Geometry check sheet. Reference: the model listing, model coordinates, mm. Face numbers are marked on the shaded views. Coordinates: 2 decimals unless noted, no trailing zeros. Order: outer loops, then holes, each group sorted by start corner. A loop starts at its lowest first (then second) coordinate and runs counter-clockwise, first axis right, second up. Notation, with made-up numbers: (1, 6.25) - (21, 6.25) arc R24 cw to (21, 40.25) - close; hole circle Ø1 at (-36, -7). An arc over 180 degrees is marked (long way). Use CSV: the item, a comma, the result in double quotes. Start each with the question number.
1) Sectioned sample at A-A, the plane y = 2.3. Record the cut outline in (x, z).
2) Sectioned sample at D-D, the plane x = 41.5. Count the separate pieces of the cut face and the enclosed holes in it, and give its area (3 significant figures).
3) Sectioned sample at C-C, the plane z = 6. Record the cut outline in (x, y), and give its area (3 significant figures).
4) Thickness scan on probe 1 along Z at (x, y) = (47, 2.15); probe 2 along Y at (x, z) = (48, 13); probe 3 along Z at (x, y) = (41, -0.4). Record the ranges inside material, lowest first. Write a range as [from, to].
5) Depth check by flat-ended pin: P1, Ø0.8, axis at y = -0.5, z = 6.5, coming from the +X side; P2, Ø17, axis at x = 36.5, z = 28.5, coming from the +Y side; P3, Ø3, axis at y = 0.5, z = 17, coming from the -X side. Enter the tip coordinate at first touch or a pass-through.
6) Sectioned sample at B-B, the plane x = 47. Record the cut outline in (y, z).
7) Draft check along Z on the marked faces 1 and 2. Enter one of: released by +Z, released by -Z, zero draft, split by the parting line, or undercut.
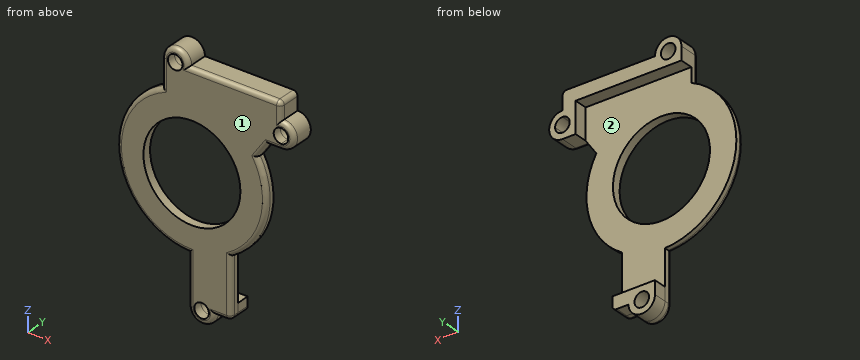
from build123d import *

# Parameters (mm, degrees)
F0_R     = 11
F1_DEPTH = 2
F2_DEPTH = 3
F3_R     = 1


with BuildPart() as f1:
    # F0 (on Front) → F1 (new body)
    with BuildSketch(Plane.XZ):
        with BuildLine():
            Line((38, 47), (38, 44))
            Line((38, 44), (62, 44))
            Line((62, 44), (62, 37))
            Line((62, 37), (65, 37))
            Line((65, 37), (65, 38.35))
            ThreePointArc((65, 38.35), (63.35, 40), (65, 41.65))
            Line((65, 41.65), (65, 43))
            Line((65, 43), (65, 47))
            Line((65, 47), (44, 47))
            Line((44, 47), (42.65, 47))
            ThreePointArc((42.65, 47), (41, 45.35), (39.35, 47))
            Line((39.35, 47), (38, 47))
        make_face()
        with BuildLine():
            ThreePointArc((44, 47), (41, 50), (38, 47))
            Line((38, 47), (39.35, 47))
            ThreePointArc((39.35, 47), (41, 48.65), (42.65, 47))
            Line((42.65, 47), (44, 47))
        make_face()
        with BuildLine():
            Line((62, 44), (38, 44))
            Line((38, 44), (38, 40.6807573628))
            ThreePointArc((38, 40.6807573628), (28.0814559879, 22.0193692019), (44, 8.1188339623))
            Line((44, 8.1188339623), (44, 0))
            Line((44, 0), (53.6880180275, 0))
            Line((53.6880180275, 0), (53.6880180275, 10.6085150677))
            ThreePointArc((53.6880180275, 10.6085150677), (61.2664808606, 20.8744813256), (59.5676963486, 33.5211130236))
            Line((59.5676963486, 33.5211130236), (62, 37))
            Line((62, 37), (62, 44))
        make_face()
        with Locations((44.8, 25.1)):
            Circle(F0_R, mode=Mode.SUBTRACT)
        with BuildLine():
            Line((53.6880180275, 0), (44, 0))
            Line((44, 0), (44, -3))
            Line((44, -3), (45.35, -3))
            ThreePointArc((45.35, -3), (47, -1.35), (48.65, -3))
            Line((48.65, -3), (50, -3))
            Line((50, -3), (53.6880180275, -3))
            Line((53.6880180275, -3), (53.6880180275, 0))
        make_face()
        with BuildLine():
            Line((45.35, -3), (44, -3))
            ThreePointArc((44, -3), (47, -6), (50, -3))
            Line((50, -3), (48.65, -3))
            ThreePointArc((48.65, -3), (47, -4.65), (45.35, -3))
        make_face()
        with BuildLine():
            Line((65, 38.35), (65, 37))
            ThreePointArc((65, 37), (68, 40), (65, 43))
            Line((65, 43), (65, 41.65))
            ThreePointArc((65, 41.65), (66.166726189, 41.166726189), (66.65, 40))
            ThreePointArc((66.65, 40), (66.166726189, 38.833273811), (65, 38.35))
        make_face()
    extrude(amount=F1_DEPTH)

    # F0 (on Front) → F2 (join)
    with BuildSketch(Plane.XZ):
        with BuildLine():
            ThreePointArc((44, 47), (41, 50), (38, 47))
            Line((38, 47), (39.35, 47))
            ThreePointArc((39.35, 47), (41, 48.65), (42.65, 47))
            Line((42.65, 47), (44, 47))
        make_face()
        with BuildLine():
            Line((38, 47), (38, 44))
            Line((38, 44), (62, 44))
            Line((62, 44), (62, 37))
            Line((62, 37), (65, 37))
            Line((65, 37), (65, 38.35))
            ThreePointArc((65, 38.35), (63.35, 40), (65, 41.65))
            Line((65, 41.65), (65, 43))
            Line((65, 43), (65, 47))
            Line((65, 47), (44, 47))
            Line((44, 47), (42.65, 47))
            ThreePointArc((42.65, 47), (41, 45.35), (39.35, 47))
            Line((39.35, 47), (38, 47))
        make_face()
        with BuildLine():
            Line((65, 38.35), (65, 37))
            ThreePointArc((65, 37), (68, 40), (65, 43))
            Line((65, 43), (65, 41.65))
            ThreePointArc((65, 41.65), (66.166726189, 41.166726189), (66.65, 40))
            ThreePointArc((66.65, 40), (66.166726189, 38.833273811), (65, 38.35))
        make_face()
        with BuildLine():
            Line((45.35, -3), (44, -3))
            ThreePointArc((44, -3), (47, -6), (50, -3))
            Line((50, -3), (48.65, -3))
            ThreePointArc((48.65, -3), (47, -4.65), (45.35, -3))
        make_face()
        with BuildLine():
            Line((53.6880180275, 0), (44, 0))
            Line((44, 0), (44, -3))
            Line((44, -3), (45.35, -3))
            ThreePointArc((45.35, -3), (47, -1.35), (48.65, -3))
            Line((48.65, -3), (50, -3))
            Line((50, -3), (53.6880180275, -3))
            Line((53.6880180275, -3), (53.6880180275, 0))
        make_face()
    extrude(amount=-F2_DEPTH)

    # F3
    f3_edges = [f1.edges().sort_by_distance(p)[0] for p in [
        (38, -2, 43.840379),
        (41, -2, 50),
        (54.5, -2, 47),
        (65, -2, 45),
        (68, -2, 40),
        (63.5, -2, 37),
        (60.783848, -2, 35.260557),
        (61.266481, -2, 20.874481),
        (44, -2, 2.559417),
        (47, -2, -6),
        (51.844009, -2, -3),
        (53.688018, -2, 3.804258),
        (65, 0.5, 47),
        (53.688018, 0.5, -3),
        (28.081456, -2, 22.019369),
    ]]
    fillet(f3_edges, radius=F3_R)


solid = f1.part
Evaluation:
1,outline,"(38, 44) - (62, 44) - (62, 37) - (65, 37) arc R3 ccw to (65, 43) - (65, 46) arc R1 ccw to (64, 47) - (44, 47) arc R3 ccw to (38, 47) - close; (44, -3) arc R3 ccw to (50, -3) - (52.69, -3) arc R1 ccw to (53.69, -2) - (53.69, 0) - (44, 0) - close; hole circle Ø3.3 at (41, 47); hole circle Ø3.3 at (47, -3); hole circle Ø3.3 at (65, 40)"
2,separate pieces,"3"
2,enclosed holes,"0"
2,area,"42.8 mm²"
3,outline,"(44, -1) arc R1 ccw to (45, -2) - (52.69, -2) arc R1 ccw to (53.69, -1) - (53.69, 0) - (44, 0) - close"
3,area,"18.9 mm²"
4,probe 1,"[-6, -4.65], [-1.35, 0], [44, 47]"
4,probe 2,"[-2, 0]"
4,probe 3,"[8.53, 14.78], [35.42, 45.35], [48.65, 50]"
5,P1,"x = 53.69"
5,P2,"y = 0"
5,P3,"x = 29.17"
6,outline,"(-2, -5) arc R1 ccw to (-1, -6) - (3, -6) - (3, -4.65) - (-2, -4.65) - close; (-2, -1.35) - (3, -1.35) - (3, 0) - (0, 0) - (0, 14.32) - (-2, 14.32) - close; (-2, 35.88) - (0, 35.88) - (0, 44) - (3, 44) - (3, 47) - (-1, 47) arc R1 ccw to (-2, 46) - close"
7,face 1,"zero draft"
7,face 2,"undercut"
